Geometry: final body of the model. Coordinates: model frame, mm. Face numbers are marked on the shaded views. Coordinates: 2 decimals unless noted, no trailing zeros. Order: outer loops, then holes, each group sorted by start corner. A loop starts at its lowest first (then second) coordinate and runs counter-clockwise, first axis right, second up. Notation, with made-up numbers: (34.25, 8.25) - (40.25, 8.25) arc R18 ccw to (40.25, 33.25) - close; hole circle Ø8 at (77, 1). An arc over 180 degrees is marked (long way). Use one line per item in the form item = value. Start each with the question number.
```python
from build123d import *

# Parameters (mm, degrees)
F0_R     = 3.175
F0_R_2   = 0.9525
F1_DEPTH = 0.635
F3_DEPTH = 0.127


with BuildPart() as f1:
    # F0 (on Top) → F1 (new body, symmetric)
    with BuildSketch(Plane.XY):
        Circle(F0_R)
        Circle(F0_R_2, mode=Mode.SUBTRACT)
    extrude(amount=F1_DEPTH, both=True)

    # F2 (on face) → F3 (cut)
    with BuildSketch(Plane(origin=(0, 0, -0.635), x_dir=(1, 0, 0), z_dir=(0, 0, -1))):
        with BuildLine():
            Line((0.0635, 0.9503809762), (0.0635, 3.1743649365))
            ThreePointArc((0.0635, 3.1743649365), (0, 3.175), (-0.0635, 3.1743649365))
            Line((-0.0635, 3.1743649365), (-0.0635, 0.9503809762))
            ThreePointArc((-0.0635, 0.9503809762), (0, 0.9525), (0.0635, 0.9503809762))
        make_face()
        with BuildLine():
            Line((-0.0635, -0.9503809762), (-0.0635, -3.1743649365))
            ThreePointArc((-0.0635, -3.1743649365), (0, -3.175), (0.0635, -3.1743649365))
            Line((0.0635, -3.1743649365), (0.0635, -0.9503809762))
            ThreePointArc((0.0635, -0.9503809762), (0, -0.9525), (-0.0635, -0.9503809762))
        make_face()
        with BuildLine():
            ThreePointArc((0.0635, -3.1743649365), (0, -3.175), (-0.0635, -3.1743649365))
            Line((-0.0635, -3.1743649365), (-0.0635, -3.81))
            Line((-0.0635, -3.81), (0.0635, -3.81))
            Line((0.0635, -3.81), (0.0635, -3.1743649365))
        make_face()
        with BuildLine():
            Line((0.0635, -0.9503809762), (0.0635, 0.9503809762))
            ThreePointArc((0.0635, 0.9503809762), (0, 0.9525), (-0.0635, 0.9503809762))
            Line((-0.0635, 0.9503809762), (-0.0635, -0.9503809762))
            ThreePointArc((-0.0635, -0.9503809762), (0, -0.9525), (0.0635, -0.9503809762))
        make_face()
        with BuildLine():
            Line((0.0635, 3.1743649365), (0.0635, 3.81))
            Line((0.0635, 3.81), (-0.0635, 3.81))
            Line((-0.0635, 3.81), (-0.0635, 3.1743649365))
            ThreePointArc((-0.0635, 3.1743649365), (0, 3.175), (0.0635, 3.1743649365))
        make_face()
    extrude(amount=-F3_DEPTH, mode=Mode.SUBTRACT)


solid = f1.part
```
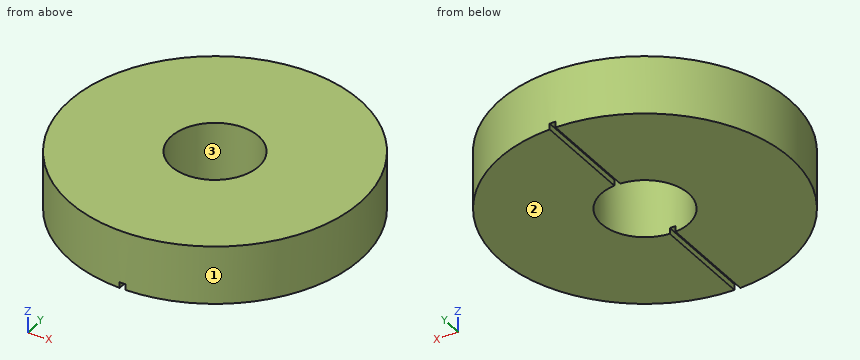
(1) Material intervals for L1, parallel to Y at x = 0, z = -0.1 (1 decimal); L2, parallel to X at y = 0.5, z = 0.2; L3, parallel to Z at x = 0, y = -1.5 (3 decimals), sorted ascending. Write a range as from..to.
(2) Contact query for a flat-ended pin moving along its axis: pin 1 Ø2 at (x, y) = (0, 0) entering from -Z (3 decimals). Output: stop coordinate, or through.
(3) Draft query along Y for the marked faces 1, 2 and 3. Return one class per face: released by +Y, released by -Y, zero draft, split by the parting line, or undercut.
(4) Cut plane A-A on y = 0. Return the cut outline in (x, z) (1 decimal).
(5) Cut plane B-B on x = 0.25. Return the cut outline in (y, z) (3 decimals).
Check sheet entries:
q1.L1 = -3.2..-1, 1..3.2
q1.L2 = -3.14..-0.81, 0.81..3.14
q1.L3 = -0.508..0.635
q2.pin_1 = -0.635
q3.face_1 = split by the parting line
q3.face_2 = zero draft
q3.face_3 = undercut
q4.outline = (-3.2, -0.6) - (-1, -0.6) - (-1, 0.6) - (-3.2, 0.6) - close; (1, -0.6) - (3.2, -0.6) - (3.2, 0.6) - (1, 0.6) - close
q5.outline = (-3.165, -0.635) - (-0.919, -0.635) - (-0.919, 0.635) - (-3.165, 0.635) - close; (0.919, -0.635) - (3.165, -0.635) - (3.165, 0.635) - (0.919, 0.635) - close
